Input: part model. Units: mm. Frame: model coordinates. A direction names the side the tool comes from. Round coordinates to 2 decimals unless told otherwise and drop trailing zeros. Order: outer loops, then holes, each group sorted by start corner. A loop starts at its lowest first (then second) coordinate and runs counter-clockwise, first axis right, second up.
Item 1: Line query: L1, parallel to Z at x = 23, y = 0.9; L2, parallel to X at y = 0.4, z = -18.35; L3, parallel to X at y = 4.15, z = -6.25. Output: solid intervals per line, ascending.
Item 2: Cut plane D-D on x = 9. Output: boundary loops of the cut face in (y, z), then the cut area to 3 significant figures.
Item 3: Cut plane B-B on z = -13.75. Output: boundary loops of the cut face in (x, y), then the cut area to 3 significant figures.
Item 4: Cut plane A-A on x = 23. Output: boundary loops of the cut face in (y, z), then the cut area to 3 significant figures.
Item 5: Reachability of faces 1 (the cylindrical face through (22.14, 0.82, -18.62)), 2 (the flat face through (2, 3, -18.25)), 3 (the flat face through (0, 3, -10)), 4 (the flat face through (2, 3, -2.25)), 5 (the flat face through (4.25, 3, -10)) from +Z, -Z, +X, -X, +Y, -Y: full face, straight path, thin tool, end or side. Return the list, or none.
Item 6: First-contact query: pin 1 (2.5 mm diameter, centred on x = 23, z = -18.35, fed in from +Y); pin 2 (1.4 mm diameter, centred on x = 23, z = -2.15, fed in from +Y); pin 3 (1.5 mm diameter, centred on y = 4, z = -6.5, fed in from -X). Flat tips, straight axial feed; report the tip coordinate or a pass-through.
Item 7: Cut plane C-C on y = 2.55. Output: boundary loops of the cut face in (x, z), then the cut area to 3 significant figures.
Item 8: Mould query, pull axis X, two halves, no side actions, for faces 6 (the flat face through (12, 0, -10)), 7 (the cylindrical face through (22.585, 0.823, -1.352)), 8 (the flat face through (25, 1, -10)). Classes: released by +X, released by -X, zero draft, split by the parting line, or undercut.
```python
from build123d import *

# Parameters (mm, degrees)
SKETCH1_W              = 25
SKETCH1_H              = 20.5
BOSS_EXTRUDE1_DEPTH    = 1.67
M1_6_CLEARANCE_HOLE1_D = 1.8
SKETCH4_W              = 4.25
SKETCH4_H              = 16
BOSS_EXTRUDE2_DEPTH    = 3.5


with BuildPart() as part:
    # Sketch1 → Boss-Extrude1 (new body)
    with BuildSketch(Plane(origin=(0, 0, 0), x_dir=(1, 0, 0), z_dir=(0, 1, 0))):
        with Locations((12.5, 10.25)):
            Rectangle(SKETCH1_W, SKETCH1_H)
    extrude(amount=BOSS_EXTRUDE1_DEPTH)

    # M1.6 Clearance Hole1 (through all)
    with Locations(Plane(origin=(0, 1.67, 0), x_dir=(1, 0, 0), z_dir=(0, 1, 0))):
        with Locations((23, 18.35), (23, 2.15)):
            Hole(M1_6_CLEARANCE_HOLE1_D / 2)

    # Sketch4 → Boss-Extrude2 (add)
    with BuildSketch(Plane(origin=(0, 1.67, 0), x_dir=(1, 0, 0), z_dir=(0, 1, 0))):
        with Locations((2.125, 10.25)):
            Rectangle(SKETCH4_W, SKETCH4_H)
    extrude(amount=BOSS_EXTRUDE2_DEPTH)


solid = part.part
```
From the geometry:
1. L1: z = -20.5 to -19.25, -17.45 to -3.05, -1.25 to 0
1. L2: x = 0 to 22.1, 23.9 to 25
1. L3: x = 0 to 4.25
2. outline: (0, -20.5) - (1.67, -20.5) - (1.67, 0) - (0, 0) - close
2. area: 34.2 mm2
3. outline: (0, 0) - (25, 0) - (25, 1.67) - (4.25, 1.67) - (4.25, 5.17) - (0, 5.17) - close
3. area: 56.6 mm2
4. outline: (0, -20.5) - (1.67, -20.5) - (1.67, -19.25) - (0, -19.25) - close; (0, -17.45) - (1.67, -17.45) - (1.67, -3.05) - (0, -3.05) - close; (0, -1.25) - (1.67, -1.25) - (1.67, 0) - (0, 0) - close
4. area: 28.2 mm2
5. face 1: +Y, -Y
5. face 2: -Z, +X, -X, +Y
5. face 3: +Z, -Z, -X, +Y, -Y
5. face 4: +Z, +X, -X, +Y
5. face 5: +Z, -Z, +X, +Y
6. pin 1: stops at y = 1.67
6. pin 2: passes through
6. pin 3: stops at x = 0
7. outline: (0, -18.25) - (4.25, -18.25) - (4.25, -2.25) - (0, -2.25) - close
7. area: 68.0 mm2
8. face 6: zero draft
8. face 7: undercut
8. face 8: released by +X
